```python
from build123d import *
from build123d.topology import SkipClean

# Parameters (mm, degrees)
SKETCH1_W           = 5
SKETCH1_H           = 2.8
SKETCH1_H_2         = 2
SKETCH1_W_2         = 15
SKETCH1_H_3         = 8.75
SKETCH1_H_4         = 9.25
SKETCH1_H_5         = 18
BOSS_EXTRUDE1_DEPTH = 4
SKETCH2_R           = 2.5
CUT_EXTRUDE1_DEPTH  = 13
SKETCH3_R           = 3
SKETCH3_R_2         = 1.6
BOSS_EXTRUDE2_DEPTH = 5
SKETCH4_R           = 2.5
CUT_EXTRUDE3_DEPTH  = 3


with BuildPart() as part:
    # Sketch1 → Boss-Extrude1 (new body)
    with BuildSketch(Plane.XY):
        with BuildLine():
            Line((-20, 0), (-15, 0))
            Line((-15, 0), (-15, 17.2))
            Line((-15, 17.2), (-20, 17.2))
            Line((-20, 17.2), (-20, 10.05))
            ThreePointArc((-20, 10.05), (-18.86862915, 9.58137085), (-18.4, 8.45))
            ThreePointArc((-18.4, 8.45), (-18.86862915, 7.31862915), (-20, 6.85))
            Line((-20, 6.85), (-20, 0))
        make_face()
        with BuildLine():
            Line((-20, 10.05), (-20, 17.2))
            Line((-20, 17.2), (-25, 17.2))
            Line((-25, 17.2), (-25, 8.45))
            Line((-25, 8.45), (-21.6, 8.45))
            ThreePointArc((-21.6, 8.45), (-21.13137085, 9.58137085), (-20, 10.05))
        make_face()
        with BuildLine():
            Line((-25, 0), (-20, 0))
            Line((-20, 0), (-20, 6.85))
            ThreePointArc((-20, 6.85), (-21.13137085, 7.31862915), (-21.6, 8.45))
            Line((-21.6, 8.45), (-25, 8.45))
            Line((-25, 8.45), (-25, 0))
        make_face()
        with Locations((-22.5, -1.4)):
            Rectangle(SKETCH1_W, SKETCH1_H)
        with Locations((-17.5, -1.4)):
            Rectangle(SKETCH1_W, SKETCH1_H)
        with BuildLine():
            Line((-20, 17.2), (-15, 17.2))
            Line((-15, 17.2), (-15, 35.2))
            Line((-15, 35.2), (-20, 35.2))
            Line((-20, 35.2), (-20, 28.05))
            ThreePointArc((-20, 28.05), (-18.86862915, 27.58137085), (-18.4, 26.45))
            ThreePointArc((-18.4, 26.45), (-18.86862915, 25.31862915), (-20, 24.85))
            Line((-20, 24.85), (-20, 17.2))
        make_face()
        with BuildLine():
            Line((-25, 17.2), (-20, 17.2))
            Line((-20, 17.2), (-20, 24.85))
            ThreePointArc((-20, 24.85), (-21.13137085, 25.31862915), (-21.6, 26.45))
            Line((-21.6, 26.45), (-25, 26.45))
            Line((-25, 26.45), (-25, 17.2))
        make_face()
        with BuildLine():
            Line((-20, 28.05), (-20, 35.2))
            Line((-20, 35.2), (-25, 35.2))
            Line((-25, 35.2), (-25, 26.45))
            Line((-25, 26.45), (-21.6, 26.45))
            ThreePointArc((-21.6, 26.45), (-21.13137085, 27.58137085), (-20, 28.05))
        make_face()
        with Locations((-17.5, 36.2)):
            Rectangle(SKETCH1_W, SKETCH1_H_2)
        with Locations((-22.5, 36.2)):
            Rectangle(SKETCH1_W, SKETCH1_H_2)
        with Locations((-7.5, 36.2)):
            Rectangle(SKETCH1_W_2, SKETCH1_H_2)
        with Locations((-32.5, 36.2)):
            Rectangle(SKETCH1_W_2, SKETCH1_H_2)
        with Locations((-32.5, 30.825)):
            Rectangle(SKETCH1_W_2, SKETCH1_H_3)
        with Locations((-32.5, 21.825)):
            Rectangle(SKETCH1_W_2, SKETCH1_H_4)
        with Locations((-7.5, 26.2)):
            Rectangle(SKETCH1_W_2, SKETCH1_H_5)
    extrude(amount=BOSS_EXTRUDE1_DEPTH)

    # Sketch2 → Cut-Extrude1 (cut)
    with BuildSketch(Plane.XY.offset(4)):
        with Locations((-35, 27.2)):
            Circle(SKETCH2_R)
        with Locations((-5, 27.2)):
            Circle(SKETCH2_R)
    extrude(amount=-CUT_EXTRUDE1_DEPTH, mode=Mode.SUBTRACT)

    # Sketch3 → Boss-Extrude2 (add)
    # profile 1 of 2: a face of its own
    with SkipClean():  # the faces are left unmerged after this step: merging them gives an invalid solid
        with BuildSketch(Plane.XY.offset(4)):
            with Locations((-20, 26.45)):
                Circle(SKETCH3_R)
            with Locations((-20, 26.45)):
                Circle(SKETCH3_R_2, mode=Mode.SUBTRACT)
        # profile 2 of 2: a face of its own
        with BuildSketch(Plane.XY.offset(4)):
            with Locations((-20, 8.45)):
                Circle(SKETCH3_R)
            with Locations((-20, 8.45)):
                Circle(SKETCH3_R_2, mode=Mode.SUBTRACT)
        extrude(amount=BOSS_EXTRUDE2_DEPTH)

    # Sketch4 → Cut-Extrude3 (cut)
    with SkipClean():  # the faces are left unmerged after this step: merging them gives an invalid solid
        with BuildSketch(Plane(origin=(0, 0, 0), x_dir=(-1, 0, 0), z_dir=(0, 0, -1))):
            with Locations((20, 26.45)):
                Circle(SKETCH4_R)
            with Locations((20, 8.45)):
                Circle(SKETCH4_R)
        extrude(amount=-CUT_EXTRUDE3_DEPTH, mode=Mode.SUBTRACT)


solid = part.part
```
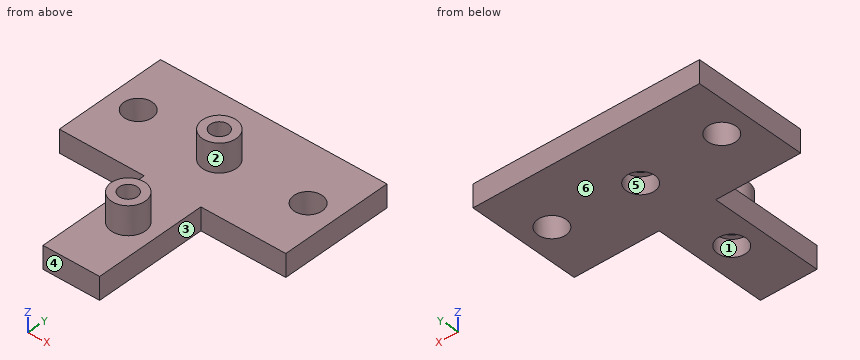
Geometry check sheet. Reference: the model listing, model coordinates, mm. Face numbers are marked on the shaded views. A direction names the side the tool comes from. Coordinates: 2 decimals unless noted, no trailing zeros. Write each loop counter-clockwise with the first axis right and the second up, starting at its lowest first coordinate (ties: lowest second). Pieces come first, ordered by that corner, then holes. Notation, with made-up numbers: M 51,35 L 90,35 A29 ccw 90,68 Z; hole C -23,-2.75 d6. An arc over 180 degrees is marked long. One line per item, written item: value. Start each with the question number.
(1) Sectioned sample at C-C, the plane z = 7.75. Enter the section's corners in (x, y).
(2) Scan lines: line 1 along Y through (x, z) = (-20, 5.7); line 2 along Y through (x, z) = (-35, 1.5); line 3 along Y through (x, z) = (-18, 1.5). Record each from-to range of solid material in increasing order. Write a range as [from, to].
(3) Sectioned sample at B-B, the plane y = 27.2. Enter the section's corners in (x, z).
(4) Sectioned sample at A-A, the plane x = -35. Enter the section's corners in (y, z).
(5) Release check for a two-part mould opening along Y. For the marked faces 4, 5 and 6 record: released by +Y, released by -Y, zero draft, split by the parting line, or undercut.
(6) Tool access check on the marked faces 1, 2 and 3. Record the directions out of +Z, -Z, +X, -X, +Y, -Y that give a thin tool (end or side, any length) a straight path to the whole face; none if there is none.
(7) Sectioned sample at D-D, the plane y = 9.5. Enter the section's corners in (x, z).
(8) Depth check by flat-ended pin: pin 1 (4.5 mm diameter, centred on x = -33, z = 2, fed in from -Y); pin 2 (4.5 mm diameter, centred on y = 7, z = 2.5, fed in from -X); pin 3 (4.5 mm diameter, centred on y = 10.5, z = 2.5, fed in from +X). Enter the tip coordinate at first touch or a pass-through.
Filled sheet:
1. outline: C -20,8.45 d6; C -20,26.45 d6; hole C -20,8.45 d3.2; hole C -20,26.45 d3.2
2. line 1: [5.45, 6.85], [10.05, 11.45], [23.45, 24.85], [28.05, 29.45]
2. line 2: [17.2, 24.7], [29.7, 37.2]
2. line 3: [-2.8, 6.95], [9.95, 24.95], [27.95, 37.2]
3. outline: M -40,0 L -37.5,0 L -37.5,4 L -40,4 Z; M -32.5,0 L -22.38,0 L -22.38,3 L -21.41,3 L -21.41,9 L -22.9,9 L -22.9,4 L -32.5,4 Z; M -18.59,3 L -17.62,3 L -17.62,0 L -7.5,0 L -7.5,4 L -17.1,4 L -17.1,9 L -18.59,9 Z; M -2.5,0 L 0,0 L 0,4 L -2.5,4 Z
4. outline: M 17.2,0 L 24.7,0 L 24.7,4 L 17.2,4 Z; M 29.7,0 L 37.2,0 L 37.2,4 L 29.7,4 Z
5. face 4: released by -Y
5. face 5: undercut
5. face 6: zero draft
6. face 1: -Z
6. face 2: +Z
6. face 3: +Z, -Z, +X, -Y
7. outline: M -25,0 L -22.27,0 L -22.27,3 L -21.21,3 L -21.21,9 L -22.81,9 L -22.81,4 L -25,4 Z; M -18.79,3 L -17.73,3 L -17.73,0 L -15,0 L -15,4 L -17.19,4 L -17.19,9 L -18.79,9 Z
8. pin 1: y = 17.2
8. pin 2: x = -25
8. pin 3: x = -15
